```python
from build123d import *

# Parameters (mm, degrees)
F0_R          = 28
F0_R_2        = 25
F1_DEPTH      = 80
F3_DEPTH      = 32.9
F3_DEPTH_BACK = 46.7
F4_R          = 4
F5_DEPTH      = 64.5
F5_DEPTH_BACK = 79.1


with BuildPart() as f1:
    # F0 (on Top) → F1 (new body)
    with BuildSketch(Plane.XY):
        Circle(F0_R)
        Circle(F0_R_2, mode=Mode.SUBTRACT)
    extrude(amount=F1_DEPTH)

    # F2 (on Front) → F3 (cut, two sides)
    with BuildSketch(Plane.XZ) as f3_sk:
        Polygon((-37.074200809, 93.2216271758), (-37.0010906232, 68.5385539477), (28, 80), align=None)
    extrude(amount=-F3_DEPTH, mode=Mode.SUBTRACT)
    extrude(f3_sk.sketch, amount=F3_DEPTH_BACK, mode=Mode.SUBTRACT)

    # F4 (on Front) → F5 (cut, two sides)
    with BuildSketch(Plane.XZ) as f5_sk:
        with Locations((0, 40)):
            Circle(F4_R)
    extrude(amount=-F5_DEPTH, mode=Mode.SUBTRACT)
    extrude(f5_sk.sketch, amount=F5_DEPTH_BACK, mode=Mode.SUBTRACT)


solid = f1.part
```
Design review of the part built by this model. Coordinates are the model's own, in mm. Give positions to 0.01 mm unless a question says otherwise; leave off trailing zeros. Order: outer loops, then holes, each group sorted by start corner. A loop starts at its lowest first (then second) coordinate and runs counter-clockwise, first axis right, second up. Notation, with made-up numbers: (-22.5, 38) -> (-6.5, 38) arc R30 cw to (-6.5, 62) -> close; hole circle Ø2 at (-10.75, 16.25). An arc over 180 degrees is marked (long way). Write item = value, one per line. Start each with the question number.
(1) We need section B-B on z = 40. Write out the cut boundary in (x, y), plus the area to 3 significant figures.
(2) We need section C-C on x = 3. Write out the cut boundary in (y, z), plus the area to 3 significant figures.
(3) For pin 1 (12 mm diameter, centred on y = -14.5, z = 15, fed in from +X); pin 2 (2 mm diameter, centred on y = 14.5, z = 9, fed in from +X); pin 3 (10 mm diameter, centred on x = -12, z = 59, fed in from -Y); pin 4 (8 mm diameter, centred on x = 20.5, y = 4, fed in from -Z), all flat-tipped, find the tip position at first contact; note any pin that passes through.
(4) We need section A-A on x = -8.5. Write out the cut boundary in (y, z), plus the area to 3 significant figures.
(5) To check wall thickness, follow line 1 along X through (y, z) = (0, 29); line 2 along Y through (x, z) = (-3, 16). State the ranges of each line that lie inside material, in increasing order.
(6) We need section D-D on z = 63. Write out the cut boundary in (x, y), plus the area to 3 significant figures.
(7) Mouldability with a two-part tool opening along Y and no side actions: class faces 1 (the face through (-11, 23, 0)), 2 (the face through (23.09, -9.58, 39.18)), 3 (the face through (25.865, -10.724, 39.44)) as +Y half, -Y half, draft (parallel to the pull), parting line (faces both ways), or undercut.
Numbers:
q1.outline = (-4, -27.71) -> (-4, -24.68) arc R25 cw to (-4, 24.68) -> (-4, 27.71) arc R28 ccw to start; (4, -27.71) arc R28 ccw to (4, 27.71) -> (4, 24.68) arc R25 cw to (4, -24.68) -> close
q1.area = 451 mm^2
q2.outline = (-27.84, 0) -> (-24.82, 0) -> (-24.82, 37.35) -> (-27.84, 37.35) -> close; (-27.84, 42.65) -> (-24.82, 42.65) -> (-24.82, 75.59) -> (-27.84, 75.59) -> close; (24.82, 0) -> (27.84, 0) -> (27.84, 37.35) -> (24.82, 37.35) -> close; (24.82, 42.65) -> (27.84, 42.65) -> (27.84, 75.59) -> (24.82, 75.59) -> close
q2.area = 425 mm^2
q3.pin_1 = 26.68
q3.pin_2 = 24.53
q3.pin_3 = -27.11
q3.pin_4 = through
q4.outline = (-26.68, 0) -> (-23.51, 0) -> (-23.51, 73.56) -> (-26.68, 73.56) -> close; (23.51, 0) -> (26.68, 0) -> (26.68, 73.56) -> (23.51, 73.56) -> close
q4.area = 466 mm^2
q5.line_1 = -28 to -25, 25 to 28
q5.line_2 = -27.84 to -24.82, 24.82 to 27.84
q6.outline = circle Ø56 at (0, 0); hole circle Ø50 at (0, 0)
q6.area = 500 mm^2
q7.face_1 = draft
q7.face_2 = undercut
q7.face_3 = parting line
